Can you work these out from the model? Positions are in its coordinate system, mm. Face numbers are marked on the shaded views. Round coordinates to 2 decimals unless told otherwise and drop trailing zeros. Order: outer loops, then holes, each group sorted by start corner. A loop starts at its lowest first (then second) coordinate and runs counter-clockwise, first axis right, second up. Notation, with made-up numbers: (85.5, 47) - (132.5, 47) arc R13 ccw to (132.5, 64) - close; hole circle Ø1 at (50, -12). An arc over 180 degrees is marked (long way). Write item = value, one per line.
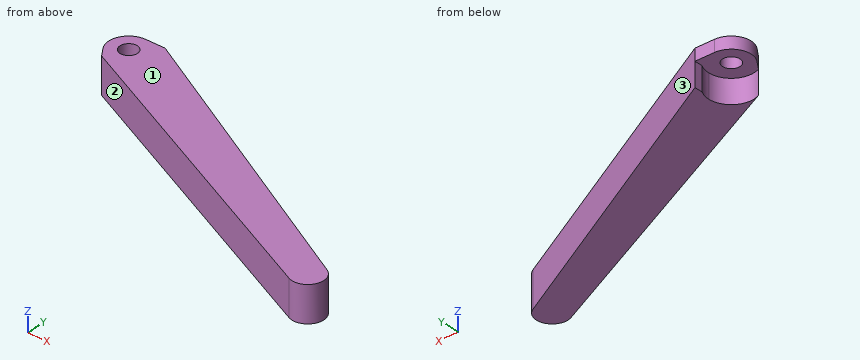
from build123d import *

# Parameters (mm, degrees)
F1_DEPTH = 9.525
F2_R     = 3.4925
F3_DEPTH = 4.7625
F5_DEPTH = 4.7625


with BuildPart() as f1:
    # F0 (on Top) → F1 (new body)
    with BuildSketch(Plane.XY):
        with BuildLine():
            Line((7.9375, 7.9375), (7.9375, 4.5076334995))
            ThreePointArc((7.9375, 4.5076334995), (8.8254506458, 2.3311128059), (9.128125, 0))
            ThreePointArc((9.128125, 0), (4.874681275, -7.7175221725), (-3.9216850064, -8.2427575923))
            Line((-3.9216850064, -8.2427575923), (124.223871162, -69.211007676))
            ThreePointArc((124.223871162, -69.211007676), (132.6511593099, -66.3960142358), (130.01461013, -57.9112053389))
            Line((130.01461013, -57.9112053389), (7.9375, 7.9375))
        make_face()
    extrude(amount=F1_DEPTH)

    # F2 (on face) → F3 (join)
    with BuildSketch(Plane.XY.offset(9.525)):
        with BuildLine():
            ThreePointArc((-6.5048555726, -4.5487097324), (2.3844931476, -7.5708717252), (7.9375, 0))
            ThreePointArc((7.9375, 0), (5.6126600757, 5.6126600757), (0, 7.9375))
            ThreePointArc((0, 7.9375), (-7.0395060107, 3.667323462), (-6.5048555726, -4.5487097324))
        make_face()
        Circle(F2_R, mode=Mode.SUBTRACT)
        with BuildLine():
            ThreePointArc((0, 7.9375), (5.6126600757, 5.6126600757), (7.9375, 0))
            ThreePointArc((7.9375, 0), (2.3844931476, -7.5708717252), (-6.5048555726, -4.5487097324))
            Line((-6.5048555726, -4.5487097324), (-3.9216850064, -8.2427575923))
            ThreePointArc((-3.9216850064, -8.2427575923), (6.6839218101, -6.2167399215), (7.9375, 4.5076334995))
            Line((7.9375, 4.5076334995), (7.9375, 7.9375))
            Line((7.9375, 7.9375), (0, 7.9375))
        make_face()
    extrude(amount=F3_DEPTH)

    # F4 (on face) → F5 (join)
    with BuildSketch(Plane.XY.offset(9.525)):
        with BuildLine():
            Line((-3.9216850064, -8.2427575923), (124.223871162, -69.211007676))
            ThreePointArc((124.223871162, -69.211007676), (132.6511593099, -66.3960142358), (130.01461013, -57.9112053389))
            Line((130.01461013, -57.9112053389), (7.9375, 7.9375))
            Line((7.9375, 7.9375), (7.9375, 4.5076334995))
            ThreePointArc((7.9375, 4.5076334995), (6.6839218101, -6.2167399215), (-3.9216850064, -8.2427575923))
        make_face()
    extrude(amount=F5_DEPTH)


solid = f1.part
(1) If we section it at A-A (z = 7.5): Write out the boundary of the cut face in (x, y).
Computed:
outline = (-3.92, -8.24) - (124.22, -69.21) arc R6.35 ccw to (130.01, -57.91) - (7.94, 7.94) - (7.94, 4.51) arc R9.13 cw to start
(2) If we section it at B-B (x = 127): Write out the boundary of the cut face in (y, z).
Computed:
outline = (-69.85, 0) - (-56.29, 0) - (-56.29, 14.29) - (-69.85, 14.29) - close
(3) Will these pins go through, and if not, where does the flat tip stop? P1, Ø4, axis at x = 0, y = 0, coming from the +Z side; P2, Ø5, axis at x = 65, z = 10, coming from the +Y side; P3, Ø2.5, axis at y = 6, z = 2.5, coming from the -X side; P4, Ø6, axis at y = -12.5, z = 4, coming from the -X side.
Computed:
P1 = through
P2 = -21.49
P3 = 7.94
P4 = -1.28
(4) If I drill on line 1 (Y direction, x = 0, z = 11.9); line 2 (Y direction, x = 64, z = 1.75); line 3 (X direction, y = -64, z = 7.5), over which ranges is the centre line in solid material (lowest first)? Write a range as from..to.
Computed:
line_1 = -10.11..-3.49, 3.49..7.94
line_2 = -40.56..-22.3
line_3 = 113.27..133.33
(5) Thinking about a two-plate mould opening in Y: for the marked faces 1, 2 and 3, which applies, +Y half, -Y half, draft (parallel to the pull), parting line (faces both ways), or undercut?
Computed:
face_1 = draft
face_2 = -Y half
face_3 = +Y half
(6) If we section it at C-C (y = -63.5): Write out the boundary of the cut face in (x, z), plus the area to 3 significant figures.
Computed:
outline = (112.22, 0) - (133.35, 0) - (133.35, 14.29) - (112.22, 14.29) - close
area = 302 mm^2
